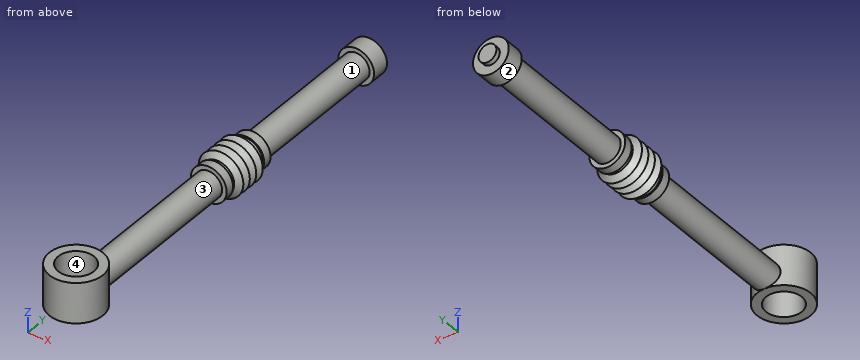
```python
from build123d import *

# Parameters (mm, degrees)
BOSS_EXTRUDE1_DEPTH                  = 4.7625
BOSS_EXTRUDE1_DEPTH_BACK             = 2.38125
SKETCH1_R                            = 4.7625
SKETCH1_R_2                          = 3.175
SKETCH2_R                            = 2.38125
BOSS_EXTRUDE2_DEPTH                  = 28.575
BOSS_EXTRUDE2_DIRECTION_2_REACH      = 13.666
BOSS_EXTRUDE2_DIRECTION_2_END_RADIUS = 4.7625
SKETCH3_W                            = 3.175
SKETCH3_H                            = 1.5875
BOSS_EXTRUDE3_START                  = 25.4
SKETCH4_R                            = 2.38125
BOSS_EXTRUDE3_DEPTH                  = 25.4
SKETCH5_R                            = 3.175
BOSS_EXTRUDE4_DEPTH                  = 3.175
SKETCH6_R                            = 1.5875
BOSS_EXTRUDE5_DEPTH                  = 0.83185


with BuildPart() as part:
    # Sketch1 → Boss-Extrude1 (new, two sides: drawn at the far end of the back side and taken through both)
    with BuildSketch(Plane.XY.offset(-BOSS_EXTRUDE1_DEPTH_BACK)):
        Circle(SKETCH1_R)
        Circle(SKETCH1_R_2, mode=Mode.SUBTRACT)
    extrude(amount=BOSS_EXTRUDE1_DEPTH + BOSS_EXTRUDE1_DEPTH_BACK)

    # Sketch2 → Boss-Extrude2 (add)
    with BuildSketch(Plane(origin=(0, 4.7625, 0), x_dir=(1, 0, 0), z_dir=(0, 1, 0))):
        with Locations(Location((0, 0, 0), (0, 0, 90.000000028))):
            Circle(SKETCH2_R)
    extrude(amount=BOSS_EXTRUDE2_DEPTH)

    # Boss-Extrude2 direction 2: up to this cylinder (the profile starts outside it)
    boss_extrude2_direction_2_end = Plane(origin=(0, 0, 0), z_dir=(0, 0, 1)) * Cylinder(BOSS_EXTRUDE2_DIRECTION_2_END_RADIUS, 37.857, mode=Mode.PRIVATE)
    # Sketch2 → Boss-Extrude2 direction 2 (add, up to the surface)
    with BuildSketch(Plane(origin=(0, 4.7625, 0), x_dir=(1, 0, 0), z_dir=(0, 1, 0)), mode=Mode.PRIVATE) as boss_extrude2_direction_2_sk1:
        with Locations(Location((0, 0, 0), (0, 0, 90.000000028))):
            Circle(SKETCH2_R)
    boss_extrude2_direction_2_tool1 = extrude(boss_extrude2_direction_2_sk1.sketch, amount=-BOSS_EXTRUDE2_DIRECTION_2_REACH, mode=Mode.PRIVATE) - boss_extrude2_direction_2_end
    add(boss_extrude2_direction_2_tool1.solids().sort_by_distance((0, 4.7625, 0))[0])
    add(boss_extrude2_direction_2_tool1.solids().sort_by_distance((0, 4.7625, 0))[1])

    # Sketch3 → Revolve1 (revolve)
    with BuildSketch(Plane(origin=(0, 0, 0), x_dir=(0, 0, -1), z_dir=(1, 0, 0)), mode=Mode.PRIVATE) as revolve1_sk:
        with Locations((-1.5875, 33.3375)):
            Rectangle(SKETCH3_W, SKETCH3_H)
        Polygon((-2.921, 34.76625), (-2.921, 34.13125), (0, 34.13125), (0, 43.33875), (-3.175, 43.33875), (-3.175, 41.75125), (-2.921, 41.75125), (-2.921, 41.11625), (-3.96875, 40.3225), (-2.921, 39.52875), (-3.96875, 38.735), (-2.921, 37.94125), (-3.96875, 37.1475), (-2.921, 36.35375), (-3.96875, 35.56), align=None)
    revolve(revolve1_sk.sketch.rotate(Axis((0, 32.54375, 0), (0, 1, 0)), 180), axis=Axis((0, 32.54375, 0), (0, 1, 0)))

    # Sketch4 → Boss-Extrude3 (add)
    with BuildSketch(Plane(origin=(0, 43.33875, 0), x_dir=(1, 0, 0), z_dir=(0, 1, 0)).offset(BOSS_EXTRUDE3_START)):
        with Locations(Location((0, 0, 0), (0, 0, 90))):
            Circle(SKETCH4_R)
    extrude(amount=-BOSS_EXTRUDE3_DEPTH)

    # Sketch5 → Boss-Extrude4 (add)
    with BuildSketch(Plane(origin=(0, 68.73875, 0), x_dir=(1, 0, 0), z_dir=(0, 1, 0))):
        with Locations(Location((0, 0, 0), (0, 0, 90))):
            Circle(SKETCH5_R)
    extrude(amount=BOSS_EXTRUDE4_DEPTH)

    # Sketch6 → Boss-Extrude5 (add)
    with BuildSketch(Plane(origin=(0, 71.91375, 0), x_dir=(1, 0, 0), z_dir=(0, 1, 0))):
        with Locations(Location((0, 0, 0), (0, 0, 270))):
            Circle(SKETCH6_R)
    extrude(amount=BOSS_EXTRUDE5_DEPTH)


solid = part.part
```
Geometry: final body of the model. Coordinates: model frame, mm. Face numbers are marked on the shaded views. A direction names the side the tool comes from. Coordinates: 2 decimals unless noted, no trailing zeros. Order: outer loops, then holes, each group sorted by start corner. A loop starts at its lowest first (then second) coordinate and runs counter-clockwise, first axis right, second up.
Item 1: Contact query for flat-ended pins moving along their axis: P1, Ø1, axis at x = -0.5, y = 62, coming from the -Z side; P2, Ø4, axis at x = -3.5, z = -2.5, coming from the +Y side; P3, Ø5, axis at x = -3, y = 58, coming from the -Z side. Output: stop coordinate, or through.
Answer:
P1: stops at z = -2.38
P2: stops at y = 71.91
P3: stops at z = -2.33
Item 2: Section query B-B (y = 24.5). Output: boundary loops of the cut face in (x, z).
Answer:
outline: circle Ø4.76 at (0, 0)
Item 3: Access query for the marked faces 3 and 4. Directions: +Z, -Z, +X, -X, +Y, -Y. A direction counts if a zero-diameter tool reaches every point of the face in a straight line with its end or side. Return the directions, or none.
Answer:
face 3: none
face 4: +Z, -Z
Item 4: Draft query along Y for the marked faces 1 and 2. Return one class per face: released by +Y, released by -Y, zero draft, split by the parting line, or undercut.
Answer:
face 1: undercut
face 2: zero draft
Item 5: Section query A-A (y = 0). Output: boundary loops of the cut face in (x, z) (1 decimal), then the cut area to 3 significant figures.
Answer:
outline: (-4.8, -2.4) - (-3.2, -2.4) - (-3.2, 4.8) - (-4.8, 4.8) - close; (3.2, -2.4) - (4.8, -2.4) - (4.8, 4.8) - (3.2, 4.8) - close
area: 22.7 mm2
Item 6: Material intervals for line 1 along Y through (x, z) = (0, 2) (1 decimal); line 2 along Y through (x, z) = (0, 0) (1 decimal); line 3 along Z through (x, y) = (4.25, -1), sorted ascending.
Answer:
line 1: y = -4.8 to -3.2, 3.2 to 71.9
line 2: y = -4.8 to -3.2, 3.2 to 72.7
line 3: z = -2.38 to 4.76
